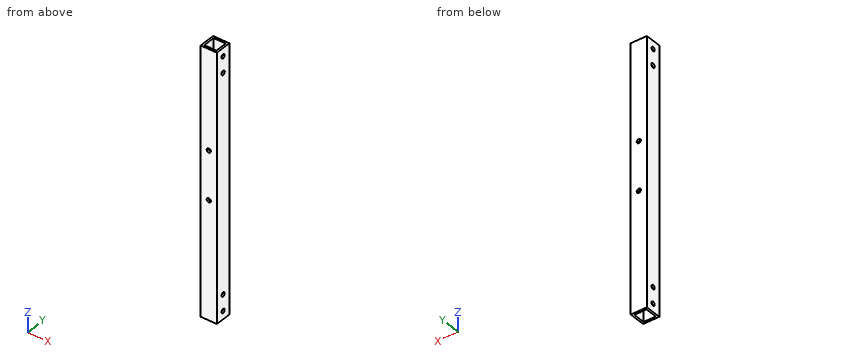
from build123d import *

# Parameters (mm, degrees)
SKETCH1_W                = 25.4
SKETCH1_H                = 25.4
SKETCH1_W_2              = 19.05
SKETCH1_H_2              = 19.05
BOSS_EXTRUDE1_DEPTH      = 415.925
F_0_257_DIAMETER_HOLE1_D = 6.5278
I_0_272_DIAMETER_HOLE1_D = 6.9088
F_0_257_DIAMETER_HOLE2_D = 6.5278


with BuildPart() as part:
    # Sketch1 → Boss-Extrude1 (new body)
    with BuildSketch(Plane.XY):
        Rectangle(SKETCH1_W, SKETCH1_H)
        Rectangle(SKETCH1_W_2, SKETCH1_H_2, mode=Mode.SUBTRACT)
    extrude(amount=BOSS_EXTRUDE1_DEPTH)

    # F (0.257) Diameter Hole1 (through all)
    with Locations(Plane(origin=(12.7, 0, 0), x_dir=(0, 0, -1), z_dir=(1, 0, 0))):
        with Locations((-403.225, 0), (-12.7, 0), (-38.1, 0)):
            Hole(F_0_257_DIAMETER_HOLE1_D / 2)

    # I (0.272) Diameter Hole1 (through all)
    with Locations(Plane(origin=(12.7, 0, 0), x_dir=(0, 0, -1), z_dir=(1, 0, 0))):
        with Locations((-377.825, 0)):
            Hole(I_0_272_DIAMETER_HOLE1_D / 2)

    # F (0.257) Diameter Hole2 (through all)
    with Locations(Plane(origin=(0, 12.7, 0), x_dir=(1, 0, 0), z_dir=(0, 1, 0))):
        with Locations((0, -184.15), (0, -260.35)):
            Hole(F_0_257_DIAMETER_HOLE2_D / 2)


solid = part.part
CAD build for the part. Positions are in the model's coordinates, mm. Give positions to 0.01 mm unless a question says otherwise; leave off trailing zeros. Write each loop counter-clockwise with the first axis right and the second up, starting at its lowest first coordinate (ties: lowest second). Pieces come first, ordered by that corner, then holes. Notation, with made-up numbers: (73, 57.25) - (78, 57.25) arc R37 ccw to (78, 95.25) - close; hole circle Ø4 at (58.25, 20). An arc over 180 degrees is marked (long way). Put each result on its own line as item: value.
(1) Drop a flat-ended pin along its axis: pin 1 Ø5 at (y, z) = (0, 38.1) entering from +X. Give the stop position or say it passes through.
Working result:
pin 1: through
(2) Wall check: L1, parallel to Y at x = -6.5, z = 191.5 (3 decimals); L2, parallel to Z at x = 0, y = 11.9 (3 decimals). Give the ranges that are in metal, low to high.
Working result:
L1: -12.7 to -9.525, 9.525 to 12.7
L2: 0 to 180.886, 187.414 to 257.086, 263.614 to 415.925
(3) Saw through at A-A (z = 57). List the corners of the cut face in (x, y) (3 decimals).
Working result:
outline: (-12.7, -12.7) - (12.7, -12.7) - (12.7, 12.7) - (-12.7, 12.7) - close; hole (-9.525, -9.525) - (9.525, -9.525) - (9.525, 9.525) - (-9.525, 9.525) - close
